```python
from build123d import *

# Parameters (mm, degrees)
F0_W      = 60.7
F0_H      = 22
F1_DEPTH  = 2
F0_W_2    = 2.65
F2_DEPTH  = 2.5
F1_FACE_W = 2
F1_FACE_H = 22
F4_DEPTH  = 30.35
F5_DEPTH  = 30.35
F6_D      = 2.5
F6_DEPTH  = 33.001
F7_D      = 2.5


with BuildPart() as f1:
    # F0 (on Front) → F1 (new body)
    with BuildSketch(Plane.XZ):
        Rectangle(F0_W, F0_H)
    extrude(amount=F1_DEPTH)

    # F0 (on Front) → F2 (join)
    with BuildSketch(Plane.XZ):
        with Locations((31.675, 0)):
            Rectangle(F0_W_2, F0_H)
        Rectangle(F0_W, F0_H)
        with Locations((-31.675, 0)):
            Rectangle(F0_W_2, F0_H)
    extrude(amount=-F2_DEPTH)

    # F3 (on Right) + F1_face (on face) → F4 (join)
    with BuildSketch(Plane.YZ):
        with BuildLine():
            ThreePointArc((0.0834241115, 0), (-2.1721045963, 2.2555287078), (-4.4276333041, 0))
            ThreePointArc((-4.4276333041, 0), (-2.1721045963, -2.2555287078), (0.0834241115, 0))
        make_face()
        with BuildLine():
            ThreePointArc((-3.4221045963, 0), (-2.1721045963, 1.25), (-0.9221045963, 0))
            ThreePointArc((-0.9221045963, 0), (-2.1721045963, -1.25), (-3.4221045963, 0))
        make_face(mode=Mode.SUBTRACT)
    with BuildSketch(Plane(origin=(-30.35, -1, 0), x_dir=(0, -1, 0), z_dir=(-1, 0, 0))):
        Rectangle(F1_FACE_W, F1_FACE_H)
    extrude(amount=F4_DEPTH, dir=(1, 0, 0))

    # F3 (on Right) → F5 (join)
    with BuildSketch(Plane.YZ):
        with BuildLine():
            ThreePointArc((0.0834241115, 0), (-2.1721045963, 2.2555287078), (-4.4276333041, 0))
            ThreePointArc((-4.4276333041, 0), (-2.1721045963, -2.2555287078), (0.0834241115, 0))
        make_face()
        with BuildLine():
            ThreePointArc((-3.4221045963, 0), (-2.1721045963, 1.25), (-0.9221045963, 0))
            ThreePointArc((-0.9221045963, 0), (-2.1721045963, -1.25), (-3.4221045963, 0))
        make_face(mode=Mode.SUBTRACT)
    extrude(amount=-F5_DEPTH)

    # F6 (through all, one way)
    with BuildSketch(Plane.YZ):
        with Locations((-2.1721045963, 0)):
            Circle(F6_D / 2)
    extrude(amount=-F6_DEPTH, mode=Mode.SUBTRACT)

    # F7 (through all)
    with Locations(Plane(origin=(0, 0, 0), x_dir=(0, 1, 0), z_dir=(-1, 0, 0))):
        with Locations((-2.1721045963, 0)):
            Hole(F7_D / 2)


solid = f1.part
```
The listing builds one solid part. Answer for the finished solid, in the listing's coordinates (mm). A direction names the side the tool comes from. Round coordinates to 2 decimals unless told otherwise and drop trailing zeros. Loops run counter-clockwise (first coordinate to the right, second up) from the corner with the lowest first, then second, coordinate; pieces in that order, holes last.
1) Given P1, Ø7, axis at x = 0, z = -8, coming from the -Y side; P2, Ø2, axis at x = -32, z = 5, coming from the -Y side; P3, Ø1, axis at x = -26, z = 2.5, coming from the -Y side, each flat-ended and moving along its own axis, determine where each tip first touches the part or whether it passes through.
Outcome:
P1: stops at y = -2
P2: stops at y = 0
P3: stops at y = -3.21
2) A cutting plane is placed at A-A on z = 4.5. Determine the outline of the cut face in (x, y).
Outcome:
outline: (-33, 0) - (-30.35, 0) - (-30.35, -2) - (30.35, -2) - (30.35, 0) - (33, 0) - (33, 2.5) - (-33, 2.5) - close
3) For faces 1 (the face through (0, -2, 7)), 2 (the face through (0, -2, -7)), 3 (the face through (-32, 0, 0)), determine the directions among +Z, -Z, +X, -X, +Y, -Y from which every point of the face is accessible in a straight line to the end or side of a thin tool.
Outcome:
face 1: +Z, +X, -X, -Y
face 2: -Z, +X, -X, -Y
face 3: +Z, -Z, -X, -Y
4) Consider line 1 (X direction, y = -0.25, z = 4.75); line 2 (Y direction, x = 14, z = -3); line 3 (Z direction, x = -28.5, y = -1.5). Determine where each line is inside the solid, lowest interval first.
Outcome:
line 1: x = -30.35 to 30.35
line 2: y = -2 to 2.5
line 3: z = -11 to -1.05, 1.05 to 11
5) A cutting plane is placed at B-B on x = -5. Determine the outline of the cut face in (y, z), plus the area to 3 significant figures.
Outcome:
outline: (-2, -11) - (2.5, -11) - (2.5, 11) - (-2, 11) - (-2, 2.25) arc R2.26 ccw (long way) to (-2, -2.25) - close; hole circle Ø2.5 at (-2.17, 0)
area: 103 mm2
